```python
from build123d import *

# Parameters (mm, degrees)
SKETCH_1_R      = 2.5
EXTRUDE_2_DEPTH = 180
EXTRUDE_3_DEPTH = 180


with BuildPart() as part:
    # 草图1 → 凸台-拉伸2 (new body)
    with BuildSketch(Plane.XY):
        with BuildLine():
            Line((3.65, 10), (8.5, 10))
            ThreePointArc((8.5, 10), (9.560660172, 9.560660172), (10, 8.5))
            Line((10, 8.5), (10, 3.65))
            Line((10, 3.65), (8.2, 3.65))
            Line((8.2, 3.65), (8.2, 5.5))
            Line((8.2, 5.5), (6.560660172, 5.5))
            Line((6.560660172, 5.5), (3.9, 2.839339828))
            Line((3.9, 2.839339828), (3.9, -2.839339828))
            Line((3.9, -2.839339828), (6.560660172, -5.5))
            Line((6.560660172, -5.5), (8.2, -5.5))
            Line((8.2, -5.5), (8.2, -3.65))
            Line((8.2, -3.65), (10, -3.65))
            Line((10, -3.65), (10, -8.5))
            ThreePointArc((10, -8.5), (9.560660172, -9.560660172), (8.5, -10))
            Line((8.5, -10), (3.65, -10))
            Line((3.65, -10), (3.65, -8.2))
            Line((3.65, -8.2), (5.5, -8.2))
            Line((5.5, -8.2), (5.5, -6.560660172))
            Line((5.5, -6.560660172), (2.839339828, -3.9))
            Line((2.839339828, -3.9), (-2.839339828, -3.9))
            Line((-2.839339828, -3.9), (-5.5, -6.560660172))
            Line((-5.5, -6.560660172), (-5.5, -8.2))
            Line((-5.5, -8.2), (-3.65, -8.2))
            Line((-3.65, -8.2), (-3.65, -10))
            Line((-3.65, -10), (-8.5, -10))
            ThreePointArc((-8.5, -10), (-9.560660172, -9.560660172), (-10, -8.5))
            Line((-10, -8.5), (-10, -3.65))
            Line((-10, -3.65), (-8.2, -3.65))
            Line((-8.2, -3.65), (-8.2, -5.5))
            Line((-8.2, -5.5), (-6.560660172, -5.5))
            Line((-6.560660172, -5.5), (-3.9, -2.839339828))
            Line((-3.9, -2.839339828), (-3.9, 2.839339828))
            Line((-3.9, 2.839339828), (-6.560660172, 5.5))
            Line((-6.560660172, 5.5), (-8.2, 5.5))
            Line((-8.2, 5.5), (-8.2, 3.65))
            Line((-8.2, 3.65), (-10, 3.65))
            Line((-10, 3.65), (-10, 8.5))
            ThreePointArc((-10, 8.5), (-9.560660172, 9.560660172), (-8.5, 10))
            Line((-8.5, 10), (-3.65, 10))
            Line((-3.65, 10), (-3.65, 8.2))
            Line((-3.65, 8.2), (-5.5, 8.2))
            Line((-5.5, 8.2), (-5.5, 6.560660172))
            Line((-5.5, 6.560660172), (-2.839339828, 3.9))
            Line((-2.839339828, 3.9), (2.839339828, 3.9))
            Line((2.839339828, 3.9), (5.5, 6.560660172))
            Line((5.5, 6.560660172), (5.5, 8.2))
            Line((5.5, 8.2), (3.65, 8.2))
            Line((3.65, 8.2), (3.65, 10))
        make_face()
        with Locations(Location((0, 0, 0), (0, 0, 180))):
            Circle(SKETCH_1_R, mode=Mode.SUBTRACT)
    extrude(amount=EXTRUDE_2_DEPTH)

    # 草图3 → 凸台-拉伸3 (add)
    with BuildSketch(Plane.XY.offset(180)):
        with BuildLine():
            Line((-8.2, 3.65), (-9.7, 3.65))
            Line((-9.7, 3.65), (-9.7, 3.3))
            ThreePointArc((-9.7, 3.3), (-9.641421356, 3.158578644), (-9.5, 3.1))
            Line((-9.5, 3.1), (-8.4, 3.1))
            ThreePointArc((-8.4, 3.1), (-8.258578644, 3.158578644), (-8.2, 3.3))
            Line((-8.2, 3.3), (-8.2, 3.65))
        make_face()
        with BuildLine():
            Line((-3.65, 9.7), (-3.65, 8.2))
            Line((-3.65, 8.2), (-3.3, 8.2))
            ThreePointArc((-3.3, 8.2), (-3.158578644, 8.258578644), (-3.1, 8.4))
            Line((-3.1, 8.4), (-3.1, 9.5))
            ThreePointArc((-3.1, 9.5), (-3.158578644, 9.641421356), (-3.3, 9.7))
            Line((-3.3, 9.7), (-3.65, 9.7))
        make_face()
        with BuildLine():
            Line((3.65, 8.2), (3.65, 9.7))
            Line((3.65, 9.7), (3.3, 9.7))
            ThreePointArc((3.3, 9.7), (3.158578644, 9.641421356), (3.1, 9.5))
            Line((3.1, 9.5), (3.1, 8.4))
            ThreePointArc((3.1, 8.4), (3.158578644, 8.258578644), (3.3, 8.2))
            Line((3.3, 8.2), (3.65, 8.2))
        make_face()
        with BuildLine():
            Line((9.7, 3.65), (8.2, 3.65))
            Line((8.2, 3.65), (8.2, 3.3))
            ThreePointArc((8.2, 3.3), (8.258578644, 3.158578644), (8.4, 3.1))
            Line((8.4, 3.1), (9.5, 3.1))
            ThreePointArc((9.5, 3.1), (9.641421356, 3.158578644), (9.7, 3.3))
            Line((9.7, 3.3), (9.7, 3.65))
        make_face()
        with BuildLine():
            Line((3.65, -9.7), (3.65, -8.2))
            Line((3.65, -8.2), (3.3, -8.2))
            ThreePointArc((3.3, -8.2), (3.158578644, -8.258578644), (3.1, -8.4))
            Line((3.1, -8.4), (3.1, -9.5))
            ThreePointArc((3.1, -9.5), (3.158578644, -9.641421356), (3.3, -9.7))
            Line((3.3, -9.7), (3.65, -9.7))
        make_face()
        with BuildLine():
            Line((-3.65, -8.2), (-3.65, -9.7))
            Line((-3.65, -9.7), (-3.3, -9.7))
            ThreePointArc((-3.3, -9.7), (-3.158578644, -9.641421356), (-3.1, -9.5))
            Line((-3.1, -9.5), (-3.1, -8.4))
            ThreePointArc((-3.1, -8.4), (-3.158578644, -8.258578644), (-3.3, -8.2))
            Line((-3.3, -8.2), (-3.65, -8.2))
        make_face()
        with BuildLine():
            Line((8.2, -3.65), (8.2, -3.3))
            ThreePointArc((8.2, -3.3), (8.258578644, -3.158578644), (8.4, -3.1))
            Line((8.4, -3.1), (9.5, -3.1))
            ThreePointArc((9.5, -3.1), (9.641421356, -3.158578644), (9.7, -3.3))
            Line((9.7, -3.3), (9.7, -3.65))
            Line((9.7, -3.65), (8.2, -3.65))
        make_face()
        with BuildLine():
            Line((-8.2, -3.65), (-8.2, -3.3))
            ThreePointArc((-8.2, -3.3), (-8.258578644, -3.158578644), (-8.4, -3.1))
            Line((-8.4, -3.1), (-9.5, -3.1))
            ThreePointArc((-9.5, -3.1), (-9.641421356, -3.158578644), (-9.7, -3.3))
            Line((-9.7, -3.3), (-9.7, -3.65))
            Line((-9.7, -3.65), (-8.2, -3.65))
        make_face()
    extrude(amount=-EXTRUDE_3_DEPTH)


solid = part.part
```
Could you check a few things on this model? Use its own coordinates, in mm. A direction names the side the tool comes from. Round coordinates to 2 decimals unless told otherwise and drop trailing zeros. Loops run counter-clockwise (first coordinate to the right, second up) from the corner with the lowest first, then second, coordinate; pieces in that order, holes last. Notation, with made-up numbers: (12, 40) - (26, 40) arc R21 ccw to (26, 71) - close; hole circle Ø8 at (86, -39). An arc over 180 degrees is marked (long way). Answer as CSV lines item,"result".
1. For pin 1 Ø2 at (y, z) = (-2.5, 156) entering from -X; pin 2 Ø2 at (x, z) = (-2.5, 41) entering from -Y; pin 3 Ø0.5 at (x, z) = (-9, 134) entering from -Y, each with a flat end and sliding along its axis, tell me the tip position at first contact or that it passes through.
Filled in:
pin 1,"stops at x = -9.7"
pin 2,"stops at y = -9.7"
pin 3,"stops at y = -9.98"
2. On a 3-axis mill with a long thin cutter (end or side, diameter ignored), from which of +Z, -Z, +X, -X, +Y, -Y can I reach the whole of each face in a straight line? I mean faces 4 (the face through (-6, -10, 89)), 5 (the face through (0, 3.9, 89)), 6 (the face through (3.9, 0, 89)). Say none if no direction works.
Filled in:
face 4,"+Z, -Z, +X, -X, -Y"
face 5,"+Z, -Z, +Y"
face 6,"+Z, -Z, +X"
3. Please list where these lines run through material, in increasing order: line 1 along Y through (x, z) = (0, 104); line 2 along Y through (x, z) = (8.5, 82.5); line 3 along X through (y, z) = (4.5, 64). Write a range as [from, to].
Filled in:
line 1,"y = [-3.9, -2.5], [2.5, 3.9]"
line 2,"y = [-10, -3.1], [3.1, 10]"
line 3,"x = [-10, -8.2], [-5.56, -3.44], [3.44, 5.56], [8.2, 10]"
4. I want a section at A-A on x = 0. List the corners of the cut face in (y, z) for me.
Filled in:
outline,"(-3.9, 0) - (-2.5, 0) - (-2.5, 180) - (-3.9, 180) - close; (2.5, 0) - (3.9, 0) - (3.9, 180) - (2.5, 180) - close"
5. We'd pull the mould along Y, two halves only. Please class faces 1 (the face through (0, -3.9, 89)), 2 (the face through (-10, -6, 89)), 3 (the face through (-3.9, 0, 89)): +Y half, -Y half, draft (parallel to the pull), parting line (faces both ways), or undercut.
Filled in:
face 1,"-Y half"
face 2,"draft"
face 3,"undercut"
